Input: part model. Units: mm. Frame: model coordinates. Round coordinates to 2 decimals unless told otherwise and drop trailing zeros. Loops run counter-clockwise (first coordinate to the right, second up) from the corner with the lowest first, then second, coordinate; pieces in that order, holes last.
1) Section B-B, the plane x = 60. Return loops of the section in (y, z), and give its area (3 significant figures).
2) Section C-C, the plane z = 0. Return loops of the section in (x, y).
3) First-contact query: pin 1 (1 mm diameter, centred on y = 4.5, z = 19.5, fed in from +X); pin 2 (1.8 mm diameter, centred on x = 20, z = 57.74, fed in from +Y); pin 3 (2 mm diameter, centred on y = 4, z = -22, fed in from -X); pin 4 (2 mm diameter, centred on y = 2.5, z = 56, fed in from +X). Flat tips, straight axial feed; report the tip coordinate or a pass-through.
4) Ray query, line 1 along Z through (x, y) = (4, 2.9); line 2 along X through (y, z) = (5.55, -45.5); line 3 along X through (y, z) = (3, 57). Return the intervals inside material, ascending.
5) Section D-D, the plane z = -34. Return loops of the section in (x, y).
6) Draft query along X for faces 1 (the face through (-41.5, 3.04, -46.25)), 2 (the face through (1, 6, -7)), 3 (the face through (22.66, 3.04, 67.45)). Return one class per face: pulls with the +X half, pulls with the -X half, needs draft (parallel to the pull), parting line crosses it, or undercut.
7) Section A-A, the plane x = 0. Return loops of the section in (y, z).
from build123d import *

# Parameters (mm, degrees)
BOSS_EXTRUDE1_DEPTH = 6
SKETCH2_R           = 3
SKETCH2_R_2         = 1.5
CUT_EXTRUDE1_DEPTH  = 7
FILLET1_R           = 5
SKETCH4_R           = 5
CUT_EXTRUDE3_DEPTH  = 7


with BuildPart() as part:
    # Sketch1 → Boss-Extrude1 (new body)
    with BuildSketch(Plane(origin=(0, 0, 0), x_dir=(1, 0, 0), z_dir=(0, 1, 0))):
        Polygon((-47.5, 54), (47.5, 54), (70.515371804, 14.13620668), (23.015371804, -68.13620668), (-23.015371804, -68.13620668), (-70.515371804, 14.13620668), align=None)
    extrude(amount=BOSS_EXTRUDE1_DEPTH)

    # Sketch2 → Cut-Extrude1 (cut, through all)
    with BuildSketch(Plane(origin=(0, 6, 0), x_dir=(1, 0, 0), z_dir=(0, 1, 0))):
        with Locations((50, 28.867513459)):
            Circle(SKETCH2_R)
        with Locations((-50, 28.867513459)):
            Circle(SKETCH2_R)
        with Locations((0, -57.735026919)):
            Circle(SKETCH2_R)
        with Locations((-20, -57.735026919)):
            Circle(SKETCH2_R_2)
        with Locations((20, -57.735026919)):
            Circle(SKETCH2_R_2)
        with Locations((0, -47.735026919)):
            Circle(SKETCH2_R_2)
        with Locations((-60, 11.547005384)):
            Circle(SKETCH2_R_2)
        with Locations((-41.339745962, 23.867513459)):
            Circle(SKETCH2_R_2)
        with Locations((-40, 46.188021535)):
            Circle(SKETCH2_R_2)
        with Locations((40, 46.188021535)):
            Circle(SKETCH2_R_2)
        with Locations((41.339745962, 23.867513459)):
            Circle(SKETCH2_R_2)
        with Locations((60, 11.547005384)):
            Circle(SKETCH2_R_2)
    extrude(amount=-CUT_EXTRUDE1_DEPTH, mode=Mode.SUBTRACT)

    # Fillet1
    fillet1_edges = [part.edges().sort_by_distance(p)[0] for p in [
        (-47.5, 3, -54),
        (47.5, 3, -54),
        (70.515371804, 3, -14.13620668),
        (23.015371804, 3, 68.13620668),
        (-23.015371804, 3, 68.13620668),
        (-70.515371804, 3, -14.13620668),
    ]]
    fillet(fillet1_edges, radius=FILLET1_R)

    # Sketch4 → Cut-Extrude3 (cut, through all)
    with BuildSketch(Plane(origin=(0, 6, 0), x_dir=(1, 0, 0), z_dir=(0, 1, 0))):
        Circle(SKETCH4_R)
    extrude(amount=-CUT_EXTRUDE3_DEPTH, mode=Mode.SUBTRACT)


solid = part.part
Final values:
1. outline: (0, -32.35) - (6, -32.35) - (6, -13.05) - (0, -13.05) - close; (0, -10.05) - (6, -10.05) - (6, 4.08) - (0, 4.08) - close
1. area: 201 mm2
2. outline: (-62.35, 0) - (-5, 0) - (-5, 6) - (-62.35, 6) - close; (5, 0) - (62.35, 0) - (62.35, 6) - (5, 6) - close
3. pin 1: stops at x = 51.38
3. pin 2: passes through
3. pin 3: stops at x = -66.55
3. pin 4: stops at x = 30.6
4. line 1: z = -54 to -3, 3 to 68.14
4. line 2: x = -52.41 to -41.33, -38.67 to 38.67, 41.33 to 52.41
4. line 3: x = -29.44 to -21.31, -18.69 to -2.91, 2.91 to 18.69, 21.31 to 29.44
5. outline: (-59.05, 0) - (59.05, 0) - (59.05, 6) - (-59.05, 6) - close
6. face 1: undercut
6. face 2: needs draft
6. face 3: pulls with the +X half
7. outline: (0, -54) - (6, -54) - (6, -5) - (0, -5) - close; (0, 5) - (6, 5) - (6, 46.24) - (0, 46.24) - close; (0, 49.24) - (6, 49.24) - (6, 54.74) - (0, 54.74) - close; (0, 60.74) - (6, 60.74) - (6, 68.14) - (0, 68.14) - close
